Check sheet for the modelled part. Datum: model origin and axes. Units: mm. Coordinates: 2 decimals unless noted, no trailing zeros. Order: outer loops, then holes, each group sorted by start corner. A loop starts at its lowest first (then second) coordinate and runs counter-clockwise, first axis right, second up. Notation, with made-up numbers: M 17.25,54.25 L 68.25,54.25 A8 ccw 68.25,64.25 Z; hole C 86.25,-16.75 d6. An arc over 180 degrees is marked long. Answer in a Markdown table with one row per item. Add a question column.
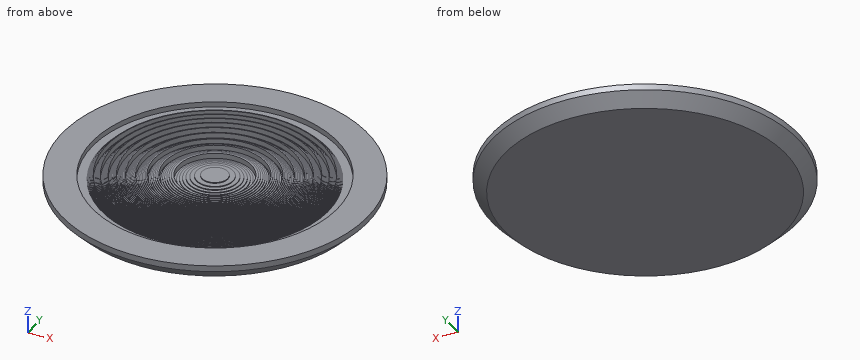
from build123d import *

# Parameters (mm, degrees)
F2_SIZE = 2


with BuildPart() as f1:
    # F0 (on Front) → F1 (revolve)
    with BuildSketch(Plane.XZ):
        Polygon((-10.558, 1.373492), (-10.558, 1.501507), (-12.7, 1.498492), (-12.7, -1.501508), (12.7, -1.501508), (12.7, 1.498492), (7.7, 1.498492), (7.7, 0.623492), (6.174, 0.623492), (6.174, 0.748492), (6.05, 0.748492), (6.05, 0.873492), (5.925, 0.873492), (5.925, 0.998492), (5.8, 0.998492), (5.8, 1.123492), (5.673, 1.123492), (5.673, 1.248492), (5.546, 1.248492), (5.546, 1.373492), (5.418, 1.373492), (5.418, 1.498492), (5.289, 1.498492), (5.289, 0.623492), (5.159, 0.623492), (5.159, 0.748492), (5.028, 0.748492), (5.028, 0.873492), (4.896, 0.873492), (4.896, 0.998492), (4.763, 0.998492), (4.763, 1.123492), (4.628998, 1.123492), (4.628998, 1.248492), (4.494, 1.248492), (4.494, 1.373492), (4.359, 1.373492), (4.359, 1.498492), (4.222, 1.498492), (4.222, 0.623492), (4.084, 0.623492), (4.084, 0.748492), (3.945, 0.748492), (3.945, 0.873492), (3.804, 0.873492), (3.804, 0.998492), (3.663, 0.998492), (3.663, 1.123492), (3.52, 1.123492), (3.52, 1.248492), (3.377, 1.248492), (3.377, 1.373492), (3.232, 1.373492), (3.232, 1.498492), (3.085, 1.498492), (3.085, 0.623492), (2.937, 0.623492), (2.937, 0.748492), (2.788, 0.748492), (2.788, 0.873492), (2.637998, 0.873492), (2.637998, 0.998492), (2.486, 0.998492), (2.486, 1.123492), (2.332, 1.123492), (2.332, 1.248492), (2.177, 1.248492), (2.177, 1.373492), (2.021, 1.373492), (2.021, 1.498492), (1.862, 1.498492), (1.862, 0.623492), (1.702, 0.623492), (1.702, 0.748492), (1.541, 0.748492), (1.541, 0.873492), (1.377, 0.873492), (1.377, 0.998492), (1.212, 0.998492), (1.212, 1.123492), (1.044, 1.123492), (1.044, 1.248492), (0.875, 1.248492), (0.875, 1.373492), (0.703, 1.373492), (0.703, 1.498492), (0.53, 1.498492), (0.53, 0.623492), (0.354, 0.623492), (0.354, 0.748492), (0.175, 0.748492), (0.175, 0.873492), (-0.006, 0.873492), (-0.006, 0.998492), (-0.189003, 0.998492), (-0.189003, 1.123492), (-0.375, 1.123492), (-0.375, 1.248492), (-0.564, 1.248492), (-0.564, 1.373492), (-0.756, 1.373492), (-0.756, 1.498492), (-0.951, 1.498492), (-0.951, 0.623492), (-1.149, 0.623492), (-1.149, 0.748492), (-1.35, 0.748492), (-1.35, 0.873492), (-1.555, 0.873492), (-1.555, 0.998492), (-1.764, 0.998492), (-1.764, 1.123492), (-1.977, 1.123492), (-1.977, 1.248492), (-2.195, 1.248492), (-2.195, 1.373492), (-2.416, 1.373492), (-2.416, 1.498492), (-2.643, 1.498492), (-2.643, 0.623492), (-2.875, 0.623492), (-2.875, 0.873492), (-3.112, 0.873492), (-3.112, 0.998492), (-3.355, 0.998492), (-3.355, 1.123492), (-3.605, 1.123492), (-3.605, 1.248492), (-3.862, 1.248492), (-3.862, 1.373492), (-4.126, 1.373492), (-4.126, 1.498492), (-4.399, 1.498492), (-4.399, 0.623492), (-4.681, 0.623492), (-4.681, 0.873492), (-4.973, 0.873492), (-4.973, 0.998492), (-5.277, 0.998492), (-5.277, 1.123492), (-5.593, 1.123492), (-5.593, 1.248492), (-5.924, 1.248492), (-5.924, 1.373492), (-6.272, 1.373492), (-6.272, 1.498492), (-6.64, 1.498492), (-6.64, 0.623492), (-7.032, 0.623492), (-7.032, 0.748492), (-7.453, 0.748492), (-7.453, 0.873492), (-7.91, 0.873492), (-7.91, 0.998492), (-8.416, 0.998492), (-8.416, 1.123492), (-8.99, 1.123492), (-8.99, 1.248492), (-9.671, 1.248492), (-9.671, 1.373492), align=None)
    revolve(axis=Axis((-12.7, 0, -0.001508), (0, 0, 1)))

    # F2
    f2_edges = [f1.edges().sort_by_distance(p)[0] for p in [
        (-38.1, 0, -1.501508),
    ]]
    chamfer(f2_edges, length=F2_SIZE)


solid = f1.part
1. Scan lines: line 1 (Z direction, x = -21.5, y = 9); line 2 (Z direction, x = -5.5, y = 5); line 3 (X direction, y = 20.5, z = 0.15). Record each from-to range of solid material in increasing order.
2. Section check A-A on z = -0.3. Enter the section's corners in (x, y).
3. Go/stop test with a flat-tipped pin: pin 1 Ø4 at (x, y) = (-23.5, 8) entering from +Z. Record where the tip stops, or that it passes through.
Result sheet:
| question | item | result |
|---|---|---|
| 1 | line 1 | -1.5 to 1 |
| 1 | line 2 | -1.5 to 1.37 |
| 1 | line 3 | -27.1 to 1.7 |
| 2 | outline | C -12.7,0 d49.2 |
| 3 | pin 1 | z = 1.5 |
